For this review, take the finished solid that the model builds, in its own axes (mm). Face numbers are marked on the shaded views. A direction names the side the tool comes from. Give positions to 0.01 mm unless a question says otherwise; leave off trailing zeros. Write each loop counter-clockwise with the first axis right and the second up, starting at its lowest first coordinate (ties: lowest second). Pieces come first, ordered by that corner, then holes. Notation, with made-up numbers: (46.5, 30) -> (80.5, 30) arc R13 ccw to (80.5, 55) -> close; hole circle Ø7 at (-29, 82.5). An arc over 180 degrees is marked (long way). Write item = value, one per line.
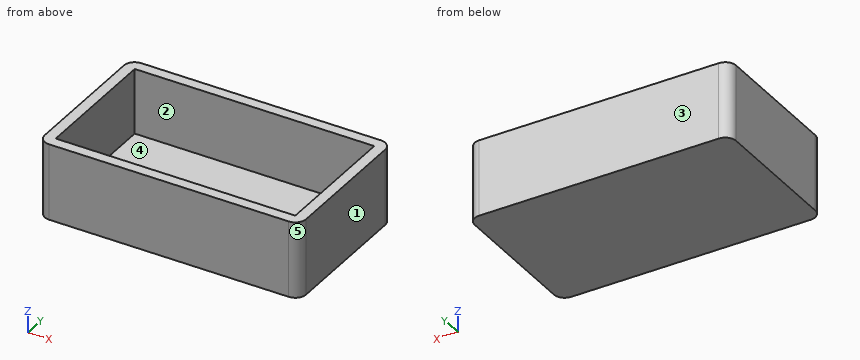
```python
from build123d import *

# Parameters (mm, degrees)
F1_DEPTH = 35
F2_T     = 5


# Not quite as in the source:
# - a shell that OpenCascade refuses in one call is made with other operations: the cavity is built on its own and cut out


with BuildPart() as f1:
    # F0 (on Top) → F1 (new body)
    with BuildSketch(Plane.XY):
        with BuildLine():
            Line((55, 35), (-55, 35))
            ThreePointArc((-55, 35), (-58.5355339059, 33.5355339059), (-60, 30))
            Line((-60, 30), (-60, -30))
            ThreePointArc((-60, -30), (-58.5355339059, -33.5355339059), (-55, -35))
            Line((-55, -35), (55, -35))
            ThreePointArc((55, -35), (58.5355339059, -33.5355339059), (60, -30))
            Line((60, -30), (60, 30))
            ThreePointArc((60, 30), (58.5355339059, 33.5355339059), (55, 35))
        make_face()
    extrude(amount=F1_DEPTH)

    # F2: shell of thickness 5, made by hand


with BuildPart() as f2_core1:
    # F2_t2: copy of F1
    add(f1.part)

    # the walls: a layer under each face that stays
    f2_faces = [f2_core1.faces().sort_by_distance(p)[0] for p in [
        (0, 35, 17.5),
        (-60, 0, 17.5),
        (0, -35, 17.5),
        (60, 0, 17.5),
        (0, 0, 0),
    ]]
    thicken(f2_faces, amount=-F2_T, mode=Mode.SUBTRACT)


with BuildPart() as f1_1:
    add(f1.part)

    # what is left inside the walls is the cavity
    f2_cavity = [f2_core1.part.solids().sort_by_distance(p)[0] for p in [
        (0, -10, 5.05),
    ]]
    add(f2_cavity, mode=Mode.SUBTRACT)


solid = f1_1.part
```
(1) Take a section at A-A (z = 10). Write out the cut boundary in (x, y).
Answers below:
outline = (-60, -30) arc R5 ccw to (-55, -35) -> (55, -35) arc R5 ccw to (60, -30) -> (60, 30) arc R5 ccw to (55, 35) -> (-55, 35) arc R5 ccw to (-60, 30) -> close; hole (-55, -30) -> (55, -30) -> (55, 30) -> (-55, 30) -> close
(2) Take a section at C-C (y = 14). Write out the cut boundary in (x, z).
Answers below:
outline = (-60, 0) -> (60, 0) -> (60, 35) -> (55, 35) -> (55, 5) -> (-55, 5) -> (-55, 35) -> (-60, 35) -> close
(3) Tool access review of the marked faces 4 and 5: name each direction out of +Z, -Z, +X, -X, +Y, -Y from which nothing blocks a thin tool from reaching the whole face with its end or side.
Answers below:
face_4 = +Z
face_5 = +Z, -Z, +X, -Y
(4) For pin 1 (1 mm diameter, centred on x = -19.5, y = 9, fed in from +Z), flat-tipped, find the tip position at first contact; note if it passes through.
Answers below:
pin_1 = 5
(5) To check wall thickness, follow probe 1 along X at (y, z) = (28.5, 10.5); probe 2 along Y at (x, z) = (5, 13); probe 3 along Z at (x, y) = (47, 24.5). State the ranges of each line that lie inside material, in increasing order.
Answers below:
probe_1 = -60 to -55, 55 to 60
probe_2 = -35 to -30, 30 to 35
probe_3 = 0 to 5
(6) The part is to be moulded in two halves that separate along Y. For the marked faces 1, 2 and 3, say which applies: released by +Y, released by -Y, zero draft, split by the parting line, or undercut.
Answers below:
face_1 = zero draft
face_2 = undercut
face_3 = released by +Y
(7) Take a section at B-B (x = 37). Write out the cut boundary in (y, z), plus the area to 3 significant figures.
Answers below:
outline = (-35, 0) -> (35, 0) -> (35, 35) -> (30, 35) -> (30, 5) -> (-30, 5) -> (-30, 35) -> (-35, 35) -> close
area = 650 mm^2
